```python
from build123d import *

# Parameters (mm, degrees)
F0_W      = 731
F0_H      = 450
F1_DEPTH  = 9
F2_W      = 731
F2_H      = 450
F2_W_2    = 722
F2_H_2    = 441
F3_DEPTH  = 4.5
F4_W      = 150
F4_H      = 9
F5_DEPTH  = 209
F6_W      = 4.5
F6_H      = 209
F7_DEPTH  = 4.5
F8_W      = 159
F8_H      = 4.5
F9_DEPTH  = 4.5
F10_W     = 25
F10_H     = 45.514172
F11_DEPTH = 9.001
F13_DEPTH = 9.001
F15_DEPTH = 9
F16_W     = 100
F16_H     = 100
F17_DEPTH = 9
F18_R     = 10
F20_DEPTH = 9
F21_W     = 6
F21_H     = 200
F22_DEPTH = 4.5
F23_W     = 146.5
F23_H     = 200
F24_DEPTH = 2


with BuildPart() as f1:
    # F0 (on Top) → F1 (new body)
    with BuildSketch(Plane.XY):
        Rectangle(F0_W, F0_H)
    extrude(amount=F1_DEPTH)

    # F2 (on face) → F3 (cut)
    with BuildSketch(Plane(origin=(0, 0, 0), x_dir=(1, 0, 0), z_dir=(0, 0, -1))):
        Rectangle(F2_W, F2_H)
        Rectangle(F2_W_2, F2_H_2, mode=Mode.SUBTRACT)
    extrude(amount=-F3_DEPTH, mode=Mode.SUBTRACT)

    # F4 (on face) → F5 (cut)
    with BuildSketch(Plane(origin=(0, 225, 0), x_dir=(-1, 0, 0), z_dir=(0, 1, 0))):
        with Locations((-210.5, 4.5)):
            Rectangle(F4_W, F4_H)
    extrude(amount=-F5_DEPTH, mode=Mode.SUBTRACT)

    # F6 (on face) → F7 (cut)
    with BuildSketch(Plane(origin=(0, 0, 0), x_dir=(1, 0, 0), z_dir=(0, 0, -1))):
        with Locations((133.25, -120.5)):
            Rectangle(F6_W, F6_H)
        with Locations((287.75, -120.5)):
            Rectangle(F6_W, F6_H)
    extrude(amount=-F7_DEPTH, mode=Mode.SUBTRACT)

    # F8 (on face) → F9 (cut)
    with BuildSketch(Plane(origin=(0, 0, 0), x_dir=(1, 0, 0), z_dir=(0, 0, -1))):
        with Locations((210.5, -13.75)):
            Rectangle(F8_W, F8_H)
    extrude(amount=-F9_DEPTH, mode=Mode.SUBTRACT)

    # F10 (on face) → F11 (cut, through all)
    with BuildSketch(Plane.XY.offset(9)):
        with BuildLine():
            Line((63, 179), (88, 179))
            ThreePointArc((88, 179), (75.5, 191.5), (63, 179))
        make_face()
        with Locations((75.5, 156.242914)):
            Rectangle(F10_W, F10_H)
        with BuildLine():
            ThreePointArc((63, 133.485828), (75.5, 120.985828), (88, 133.485828))
            Line((88, 133.485828), (63, 133.485828))
        make_face()
    extrude(amount=-F11_DEPTH, mode=Mode.SUBTRACT)

    # F12 (on face) → F13 (cut, through all)
    with BuildSketch(Plane.XY.offset(9)):
        with BuildLine():
            Line((-183, -36.5), (-258, -36.5))
            ThreePointArc((-258, -36.5), (-270.5, -49), (-258, -61.5))
            Line((-258, -61.5), (-183, -61.5))
            ThreePointArc((-183, -61.5), (-170.5, -49), (-183, -36.5))
        make_face()
        with BuildLine():
            Line((-68, -36.5), (-143, -36.5))
            ThreePointArc((-143, -36.5), (-155.5, -49), (-143, -61.5))
            Line((-143, -61.5), (-68, -61.5))
            ThreePointArc((-68, -61.5), (-55.5, -49), (-68, -36.5))
        make_face()
    extrude(amount=-F13_DEPTH, mode=Mode.SUBTRACT)

    # F14 (on face) → F15 (cut, through all)
    with BuildSketch(Plane.XY.offset(9)):
        with BuildLine():
            ThreePointArc((-270.5, 175.5), (-283, 188), (-295.5, 175.5))
            Line((-295.5, 175.5), (-295.5, 100.5))
            ThreePointArc((-295.5, 100.5), (-283, 88), (-270.5, 100.5))
            Line((-270.5, 100.5), (-270.5, 175.5))
        make_face()
    extrude(amount=-F15_DEPTH, mode=Mode.SUBTRACT)

    # F16 (on face) → F17 (cut, through all)
    with BuildSketch(Plane(origin=(0, 0, 0), x_dir=(1, 0, 0), z_dir=(0, 0, -1))):
        with Locations((-29.5, -104)):
            Rectangle(F16_W, F16_H)
    extrude(amount=-F17_DEPTH, mode=Mode.SUBTRACT)

    # F18
    f18_edges = [f1.edges().sort_by_distance(p)[0] for p in [
        (20.5, 154, 4.5),
        (-79.5, 154, 4.5),
        (-79.5, 54, 4.5),
        (20.5, 54, 4.5),
    ]]
    fillet(f18_edges, radius=F18_R)

    # F19 (on face) → F20 (cut, through all)
    with BuildSketch(Plane.XY.offset(9)):
        with BuildLine():
            ThreePointArc((258, -170.5), (270.5, -158), (258, -145.5))
            Line((258, -145.5), (183, -145.5))
            ThreePointArc((183, -145.5), (170.5, -158), (183, -170.5))
            Line((183, -170.5), (258, -170.5))
        make_face()
    extrude(amount=-F20_DEPTH, mode=Mode.SUBTRACT)

    # F21 (on face) → F22 (cut)
    with BuildSketch(Plane(origin=(0, 0, 0), x_dir=(1, 0, 0), z_dir=(0, 0, -1))):
        with Locations((-36, 120.5)):
            Rectangle(F21_W, F21_H)
        with Locations((116.5, 120.5)):
            Rectangle(F21_W, F21_H)
    extrude(amount=-F22_DEPTH, mode=Mode.SUBTRACT)

    # F23 (on face) → F24 (cut)
    with BuildSketch(Plane(origin=(0, 0, 0), x_dir=(1, 0, 0), z_dir=(0, 0, -1))):
        with Locations((40.25, 120.5)):
            Rectangle(F23_W, F23_H)
    extrude(amount=-F24_DEPTH, mode=Mode.SUBTRACT)


solid = f1.part
```
Source: CAD feature listing. Evaluate the final solid. Frame: model axes, mm. A direction names the side the tool comes from. Round coordinates to 2 decimals unless told otherwise and drop trailing zeros. Write each loop counter-clockwise with the first axis right and the second up, starting at its lowest first coordinate (ties: lowest second). Pieces come first, ordered by that corner, then holes. Notation, with made-up numbers: M 27,54 L 39,54 A20 ccw 39,75 Z; hole C 46.5,-18.75 d2. An arc over 180 degrees is marked long. Answer as a JSON object with one key per item and string values. Group by question number.
(1) Reachability of faces 1 (the flat face through (-5, 3, 9)), 2 (the flat face through (39, -122, 2)) from +Z, -Z, +X, -X, +Y, -Y: full face, straight path, thin tool, end or side. Return the list, or none.
(2) First-contact query: pin 1 (2 mm diameter, centred on x = 231.5, z = 6, fed in from +Y); pin 2 (1.3 mm diameter, centred on y = 166.5, z = 2.5, fed in from -X); pin 3 (1.3 mm diameter, centred on x = -235, z = 3, fed in from -Y). Flat tips, straight axial feed; report the tip coordinate or a pass-through.
(3) Section query B-B on x = 75.5. Output: boundary loops of the cut face in (y, z), then the cut area to 3 significant figures.
(4) Section query C-C on y = 164. Output: boundary loops of the cut face in (x, z), then the cut area to 3 significant figures.
(5) Section query A-A on y = -49. Output: boundary loops of the cut face in (x, z).
(6) Section query D-D on y = 30. Output: boundary loops of the cut face in (x, z), then the cut area to 3 significant figures.
(7) Ray query, line 1 (X direction, y = -95, z = 4); line 2 (X direction, y = 72, z = 2.75); line 3 (X direction, y = 46, z = 1.25). Return the intervals inside material, ascending. Write a range as [from, to].
Computed values:
{
 "1": {"face 1": "+Z, +X, -X, +Y, -Y", "face 2": "-Z, -Y"},
 "2": {"pin 1": "y = 16", "pin 2": "x = -361", "pin 3": "y = -220.5"},
 "3": {"outline": "M -225,4.5 L -220.5,4.5 L -220.5,2 L -20.5,2 L -20.5,0 L 120.99,0 L 120.99,9 L -225,9 Z; M 191.5,0 L 220.5,0 L 220.5,4.5 L 225,4.5 L 225,9 L 191.5,9 Z", "area": "2,970 mm^2"},
 "4": {"outline": "M -365.5,4.5 L -361,4.5 L -361,0 L -295.5,0 L -295.5,9 L -365.5,9 Z; M -270.5,0 L 63,0 L 63,9 L -270.5,9 Z; M 88,0 L 131,0 L 131,4.5 L 135.5,4.5 L 135.5,9 L 88,9 Z; M 285.5,4.5 L 290,4.5 L 290,0 L 361,0 L 361,4.5 L 365.5,4.5 L 365.5,9 L 285.5,9 Z", "area": "4,700 mm^2"},
 "5": {"outline": "M -365.5,4.5 L -361,4.5 L -361,0 L -270.5,0 L -270.5,9 L -365.5,9 Z; M -170.5,0 L -155.5,0 L -155.5,9 L -170.5,9 Z; M -55.5,0 L -39,0 L -39,4.5 L -33,4.5 L -33,2 L 113.5,2 L 113.5,4.5 L 119.5,4.5 L 119.5,0 L 361,0 L 361,4.5 L 365.5,4.5 L 365.5,9 L -55.5,9 Z"},
 "6": {"outline": "M -365.5,4.5 L -361,4.5 L -361,0 L 131,0 L 131,4.5 L 135.5,4.5 L 135.5,9 L -365.5,9 Z; M 285.5,4.5 L 290,4.5 L 290,0 L 361,0 L 361,4.5 L 365.5,4.5 L 365.5,9 L 285.5,9 Z", "area": "5,150 mm^2"},
 "7": {"line 1": "[-361, -39], [-33, 113.5], [119.5, 361]", "line 2": "[-361, -79.5], [20.5, 131], [290, 361]", "line 3": "[-361, 131], [290, 361]"}
}
